```python
from build123d import *

# Parameters (mm, degrees)
RESSALTO_EXTRUS_O1_DEPTH = 10
CORTE_EXTRUS_O1_START    = -10
CORTE_EXTRUS_O1_DEPTH    = 8
FILETE1_R                = 3


with BuildPart() as part:
    # Esboço1 → Ressalto-extrusão1 (new body)
    with BuildSketch(Plane.XY):
        with BuildLine():
            Line((0, 8.485281374), (0, 53.514718626))
            ThreePointArc((0, 53.514718626), (-0.456722805, 55.81081922), (-1.757359313, 57.757359313))
            Line((-1.757359313, 57.757359313), (-4.242640687, 60.242640687))
            ThreePointArc((-4.242640687, 60.242640687), (-6.18918078, 61.543277195), (-8.485281374, 62))
            Line((-8.485281374, 62), (-57.7, 62))
            Line((-57.7, 62), (-57.7, 58.75))
            ThreePointArc((-57.7, 58.75), (-55.923006732, 53.82983829), (-51.412210065, 51.180610148))
            Line((-51.412210065, 51.180610148), (-35.972254096, 48.3))
            Line((-35.972254096, 48.3), (-24.993325909, 48.3))
            ThreePointArc((-24.993325909, 48.3), (-19.124339626, 45.868986284), (-16.693325909, 40))
            Line((-16.693325909, 40), (-16.693325909, 19.25))
            ThreePointArc((-16.693325909, 19.25), (-19.124339626, 13.381013716), (-24.993325909, 10.95))
            Line((-24.993325909, 10.95), (-25, 10.95))
            ThreePointArc((-25, 10.95), (-30.444722215, 8.694722215), (-32.7, 3.25))
            Line((-32.7, 3.25), (-32.7, 0))
            Line((-32.7, 0), (-8.485281374, 0))
            ThreePointArc((-8.485281374, 0), (-6.18918078, 0.456722805), (-4.242640687, 1.757359313))
            Line((-4.242640687, 1.757359313), (-1.757359313, 4.242640687))
            ThreePointArc((-1.757359313, 4.242640687), (-0.456722805, 6.18918078), (0, 8.485281374))
        make_face()
    extrude(amount=RESSALTO_EXTRUS_O1_DEPTH)

    # Esboço3 → Corte-extrusão1 (cut)
    with BuildSketch(Plane.XY.offset(10).offset(CORTE_EXTRUS_O1_START)):
        Polygon((-16.693325909, 41), (-12.193325909, 41), (-12.193325909, 21), (-16.693325909, 21), (-18.193325909, 21), (-18.193325909, 41), align=None)
    extrude(amount=CORTE_EXTRUS_O1_DEPTH, mode=Mode.SUBTRACT)

    # Filete1
    filete1_edges = [part.edges().sort_by_distance(p)[0] for p in [
        (-12.193325909, 21, 4),
        (-12.193325909, 41, 4),
    ]]
    fillet(filete1_edges, radius=FILETE1_R)


solid = part.part
```
The model under review builds one solid part; all positions refer to its coordinate system, in mm. A direction names the side the tool comes from. Give positions to 0.01 mm unless a question says otherwise; leave off trailing zeros. Write each loop counter-clockwise with the first axis right and the second up, starting at its lowest first coordinate (ties: lowest second). Pieces come first, ordered by that corner, then holes.
(1) Consider section C-C, the plane x = -3.5. Give the boundary of the cut face in (y, z), and give its area (3 significant figures).
(2) To check wall thickness, follow L1, parallel to Y at x = -16.5, z = 1; L2, parallel to Z at x = -15, y = 36; L3, parallel to Y at x = -22.5, z = 9.25. State the ranges of each line that lie inside material, in increasing order.
(3) The part is to be moulded in two halves that separate along Y. For faces 4 (the cylindrical face through (-55.97, 53.89, 4.93)), 5 (the cylindrical face through (-19.06, 13.446, 4.93)), 6 (the cylindrical face through (-0.444, 55.78, 4.93)), say which applies: released by +Y, released by -Y, zero draft, split by the parting line, or undercut.
(4) For P1, Ø3.5, axis at y = 2, z = 4.5, coming from the -X side; P2, Ø2.5, axis at x = -14, y = 31.5, coming from the -Z side; P3, Ø2, axis at y = 36.5, z = 5.5, coming from the -X side, all flat-tipped, find the tip position at first contact; note any pin that passes through.
(5) Tool access review of faces 1 (the flat face through (-43.8, 49.76, 4.93)), 2 (the cylindrical face through (-13.05, 40.1, 4.06)), 3 (the cylindrical face through (-19.189, 45.933, 4.93)): name each direction out of +Z, -Z, +X, -X, +Y, -Y from which nothing blocks a thin tool from reaching the whole face with its end or side.
(6) Consider section B-B, the plane y = 29.5. Give the boundary of the cut face in (x, z).
Returned:
1. outline: (2.5, 0) - (59.5, 0) - (59.5, 10) - (2.5, 10) - close
1. area: 570 mm2
2. L1: y = 0 to 21, 41 to 62
2. L2: z = 8 to 10
2. L3: y = 0 to 11.33, 47.92 to 62
3. face 4: released by -Y
3. face 5: undercut
3. face 6: released by +Y
4. P1: stops at x = -32.7
4. P2: stops at z = 8
4. P3: stops at x = -12.19
5. face 1: +Z, -Z, -X, -Y
5. face 2: -Z, -X
5. face 3: +Z, -Z, -X
6. outline: (-16.69, 8) - (-12.19, 8) - (-12.19, 0) - (0, 0) - (0, 10) - (-16.69, 10) - close
